The figure shows three views and two pictorial views of one solid part (mm, origin at its lowest corner). Answer the questions. A direction names the side the tool comes from. Give positions to 0.01 mm unless a question says otherwise; leave off trailing zeros. Order: outer loops, then holes, each group sorted by start corner. A loop starts at its lowest first (then second) coordinate and runs counter-clockwise, first axis right, second up. Notation, with made-up numbers: (66, -36) - (83, -36) arc R17 cw to (83, -7) - close; hole circle Ø9 at (6, 78). An arc over 180 degrees is marked (long way). Use a Markdown table: item, result. Add a question column.
1. A cutting plane is placed at D-D on x = 10.5. Determine the outline of the cut face in (y, z), and give its area (3 significant figures).
2. For a pull along Y with two mould halves and no side action, classify the marked faces 3, 4, 5 and 6 as released by +Y, released by -Y, zero draft, split by the parting line, or undercut.
3. A cutting plane is placed at A-A on z = 2.35. Determine the outline of the cut face in (x, y).
4. A cutting plane is placed at C-C on x = 18.25. Determine the outline of the cut face in (y, z), and give its area (3 significant figures).
5. A cutting plane is placed at B-B on y = 3.4. Determine the outline of the cut face in (x, z), and give its area (3 significant figures).
6. Consider L1, parallel to X at y = 4.1, z = 1.7; L2, parallel to Y at x = 16.75, z = 0.6; L3, parallel to Z at x = 18, y = 2.75. Determine where each line is inside the solid, lowest interval first.
7. Which of the six approach directions +Z, -Z, +X, -X, +Y, -Y give full straight-line access (tool end or side, diameter ignored) to the marked faces 1 and 2?
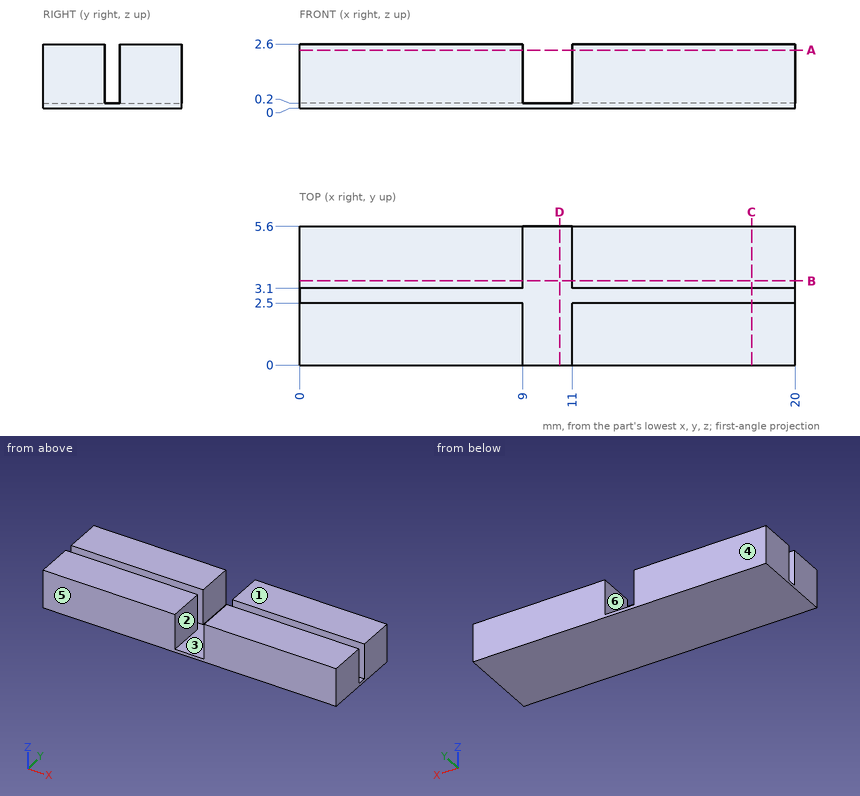
Output values:
| question | item | result |
|---|---|---|
| 1 | outline | (0, 0) - (5.6, 0) - (5.6, 0.2) - (0, 0.2) - close |
| 1 | area | 1.12 mm² |
| 2 | face 3 | undercut |
| 2 | face 4 | released by +Y |
| 2 | face 5 | released by -Y |
| 2 | face 6 | zero draft |
| 3 | outline | (0, 0) - (9, 0) - (9, 2.5) - (0, 2.5) - close; (0, 3.1) - (9, 3.1) - (9, 5.6) - (0, 5.6) - close; (11, 0) - (20, 0) - (20, 2.5) - (11, 2.5) - close; (11, 3.1) - (20, 3.1) - (20, 5.6) - (11, 5.6) - close |
| 4 | outline | (0, 0) - (5.6, 0) - (5.6, 2.6) - (3.1, 2.6) - (3.1, 0.2) - (2.5, 0.2) - (2.5, 2.6) - (0, 2.6) - close |
| 4 | area | 13.1 mm² |
| 5 | outline | (0, 0) - (20, 0) - (20, 2.6) - (11, 2.6) - (11, 0.2) - (9, 0.2) - (9, 2.6) - (0, 2.6) - close |
| 5 | area | 47.2 mm² |
| 6 | L1 | 0 to 9, 11 to 20 |
| 6 | L2 | 0 to 2.5, 3.1 to 5.6 |
| 6 | L3 | 0 to 0.2 |
| 7 | face 1 | +Z, +X, -X, +Y, -Y |
| 7 | face 2 | +Z, +Y, -Y |
